For this review, take the finished solid that the model builds, in its own axes (mm). A direction names the side the tool comes from. Coordinates: 2 decimals unless noted, no trailing zeros. Order: outer loops, then holes, each group sorted by start corner. A loop starts at its lowest first (then second) coordinate and runs counter-clockwise, first axis right, second up.
Autodesk Inventor part; units mm, degrees
ref_plane "YZ Plane" through (0, 0, 0) normal (1, 0, 0) x (0, 1, 0)
ref_plane "XZ Plane" through (0, 0, 0) normal (0, 1, 0) x (-1, 0, 0)
ref_plane "XY Plane" through (0, 0, 0) normal (0, 0, 1) x (1, 0, 0)
sketch "Sketch1" plane through (0, 0, 0) normal (0, 0, 1) x (1, 0, 0)
  circle A0 centre (0, 0) radius 2.5
  dimension "d0" = 5
extrude "Extrusion1" add sketch "Sketch1" along normal blind 160
sketch "Sketch2" plane through (0, 0, 160) normal (0, 0, 1) x (1, 0, 0)
  circle A0 centre (0, 0) radius 2.5
  circle A1 centre (0, 0) radius 1
  dimension "d3" = 2
extrude "Extrusion2" add sketch "Sketch2" along normal blind 3 contours A1
sketch "Sketch3" plane through (0, 0, 0) normal (0, 0, -1) x (-1, 0, 0)
  circle A0 centre (0, 0) radius 1
  dimension "d6" = 2
extrude "Extrusion3" add sketch "Sketch3" along normal blind 3
properties part number "Bone-16cm"
1. Take a section at C-C, the plane z = 28. Give the boundary of the cut face in (x, y), plus the area to 3 significant figures.
Answer below:
outline: circle Ø5 at (0, 0)
area: 19.6 mm2
2. Clearance check with flat-ended pins moving along their axes: pin 1 Ø3 at (x, z) = (1.5, 14.5) entering from +Y; pin 2 Ø1.5 at (y, z) = (1, 55) entering from +X. State where each tip first meets the part, or that it passes through.
Answer below:
pin 1: stops at y = 2.5
pin 2: stops at x = 2.49
3. To check wall thickness, follow L1, parallel to Z at x = -1, y = 2; L2, parallel to X at y = -0.1, z = 120; L3, parallel to Y at x = -2.3, z = 64.5. State the ranges of each line that lie inside material, in increasing order.
Answer below:
L1: z = 0 to 160
L2: x = -2.5 to 2.5
L3: y = -0.98 to 0.98
4. Take a section at A-A, the plane y = 0. Give the boundary of the cut face in (x, z).
Answer below:
outline: (-2.5, 0) - (-1, 0) - (-1, -3) - (1, -3) - (1, 0) - (2.5, 0) - (2.5, 160) - (1, 160) - (1, 163) - (-1, 163) - (-1, 160) - (-2.5, 160) - close
5. Machinability: for faces 1 (the face through (1, -1, 160)), 2 (the face through (1, -1, 0)), 3 (the face through (-0.54, 2.44, 78.88)), which of the approach directions +Z, -Z, +X, -X, +Y, -Y give a long, thin tool a straight path to every point of the face, cutting with its end or side? Answer none if there is none.
Answer below:
face 1: +Z
face 2: -Z
face 3: +Z, -Z
